```python
from build123d import *

# Parameters (mm, degrees)
CROQUIS2_R              = 20
SALIENTE_EXTRUIR1_DEPTH = 9.8
CROQUIS3_W              = 5
CROQUIS3_H              = 10
SALIENTE_EXTRUIR2_DEPTH = 5
CROQUIS4_R              = 1
CORTAR_EXTRUIR1_DEPTH   = 38.084902589


with BuildPart() as part:
    # Croquis2 → Saliente-Extruir1 (new body)
    with BuildSketch(Plane(origin=(0, 0, 0), x_dir=(1, 0, 0), z_dir=(0, 1, 0))):
        with Locations(Location((0, 0, 0), (0, 0, 270))):
            Circle(CROQUIS2_R)
    extrude(amount=SALIENTE_EXTRUIR1_DEPTH)

    # Croquis3 → Saliente-Extruir2 (add)
    with BuildSketch(Plane(origin=(0, 9.8, 0), x_dir=(1, 0, 0), z_dir=(0, 1, 0))):
        with Locations((5, 0)):
            Rectangle(CROQUIS3_W, CROQUIS3_H)
        with Locations((-5, 0)):
            Rectangle(CROQUIS3_W, CROQUIS3_H)
    extrude(amount=SALIENTE_EXTRUIR2_DEPTH)

    # Croquis4 → Cortar-Extruir1 (cut, through all)
    with BuildSketch(Plane.ZY.offset(7.5)):
        with Locations((0, 12.3)):
            Circle(CROQUIS4_R)
    extrude(amount=-CORTAR_EXTRUIR1_DEPTH, mode=Mode.SUBTRACT)


solid = part.part
```
The model under review builds one solid part; all positions refer to its coordinate system, in mm. A direction names the side the tool comes from. Round coordinates to 2 decimals unless told otherwise and drop trailing zeros. Loops run counter-clockwise (first coordinate to the right, second up) from the corner with the lowest first, then second, coordinate; pieces in that order, holes last.
Item 1: Take a section at A-A (z = 0). Write out the cut boundary in (x, y).
Determined:
outline: (-20, 0) - (20, 0) - (20, 9.8) - (7.5, 9.8) - (7.5, 11.3) - (2.5, 11.3) - (2.5, 9.8) - (-2.5, 9.8) - (-2.5, 11.3) - (-7.5, 11.3) - (-7.5, 9.8) - (-20, 9.8) - close; (-7.5, 13.3) - (-2.5, 13.3) - (-2.5, 14.8) - (-7.5, 14.8) - close; (2.5, 13.3) - (7.5, 13.3) - (7.5, 14.8) - (2.5, 14.8) - close
Item 2: Mouldability with a two-part tool opening along Z and no side actions: class faces 6 (the face through (5, 12, -5)), 7 (the face through (5, 14.8, 0)), 8 (the face through (4.965, 11.324, -0.217)), 9 (the face through (-19.524, 4.831, -4.336)) as released by +Z, released by -Z, zero draft, split by the parting line, or undercut.
Determined:
face 6: released by -Z
face 7: zero draft
face 8: undercut
face 9: split by the parting line
Item 3: Take a section at D-D (x = 0). Write out the cut boundary in (y, z), then the cut area to 3 significant figures.
Determined:
outline: (0, -20) - (9.8, -20) - (9.8, 20) - (0, 20) - close
area: 392 mm2
Item 4: Clearance check with flat-ended pins moving along their axes: pin 1 Ø2.5 at (y, z) = (12.3, 0) entering from +X; pin 2 Ø1 at (x, y) = (-15, 6) entering from -Z (3 decimals); pin 3 Ø4 at (y, z) = (11.5, 0.5) entering from +X; pin 4 Ø6 at (x, z) = (-1, -13) entering from -Y. State where each tip first meets the part, or that it passes through.
Determined:
pin 1: stops at x = 7.5
pin 2: stops at z = -13.775
pin 3: stops at x = 20
pin 4: stops at y = 0
Item 5: For line 1 (Y direction, x = -5, z = 0); line 2 (Y direction, x = -8, z = -3); line 3 (Z direction, x = 7, y = 10.25), list the stretches that pass through material, from the lowest coordinate up.
Determined:
line 1: y = 0 to 11.3, 13.3 to 14.8
line 2: y = 0 to 9.8
line 3: z = -5 to 5
Item 6: Take a section at B-B (y = 12.3). Write out the cut boundary in (x, z).
Determined:
outline: (-7.5, -5) - (-2.5, -5) - (-2.5, -1) - (-7.5, -1) - close; (-7.5, 1) - (-2.5, 1) - (-2.5, 5) - (-7.5, 5) - close; (2.5, -5) - (7.5, -5) - (7.5, -1) - (2.5, -1) - close; (2.5, 1) - (7.5, 1) - (7.5, 5) - (2.5, 5) - close
Item 7: Take a section at C-C (x = -6). Write out the cut boundary in (y, z), then the cut area to 3 significant figures.
Determined:
outline: (0, -19.08) - (9.8, -19.08) - (9.8, -5) - (14.8, -5) - (14.8, 5) - (9.8, 5) - (9.8, 19.08) - (0, 19.08) - close; hole circle Ø2 at (12.3, 0)
area: 421 mm2
Item 8: For faces 1 (the face through (-2.5, 11, 0)), 2 (the face through (7.5, 11, 0)), 3 (the face through (-5, 12, -5)), 4 (the face through (-5, 12, 5)), 5 (the face through (-7.5, 11, 0)), list the 3-axis set-ups (+Z, -Z, +X, -X, +Y, -Y) from which the entire face can be reached by the end or side of a thin tool; tool diameter is ignored.
Determined:
face 1: +Z, -Z, +Y
face 2: +Z, -Z, +X, +Y
face 3: -Z, +X, -X, +Y
face 4: +Z, +X, -X, +Y
face 5: +Z, -Z, -X, +Y
